The figure shows three views and two pictorial views of one solid part (mm, origin at its lowest corner). Answer the questions. A direction names the side the tool comes from. Round coordinates to 2 decimals unless told otherwise and drop trailing zeros. Order: outer loops, then holes, each group sorted by start corner. A loop starts at its lowest first (then second) coordinate and runs counter-clockwise, first axis right, second up. Notation, with made-up numbers: M 0.5,3.5 L 8.5,3.5 A21 cw 8.5,9.5 Z; hole C 3,-7 d9. An arc over 180 degrees is marked long. Answer as CSV lines item,"result".
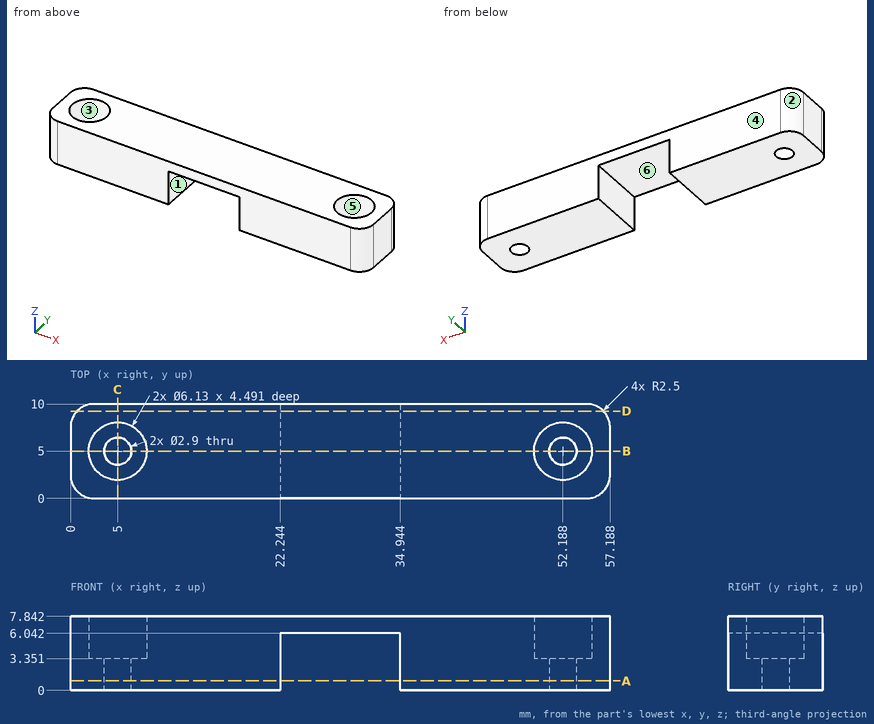
Item 1: A cutting plane is placed at C-C, the plane x = 5. Determine the outline of the cut face in (y, z) (3 decimals).
Ans:
outline,"M 0,0 L 3.55,0 L 3.55,3.351 L 1.935,3.351 L 1.935,7.842 L 0,7.842 Z; M 6.45,0 L 10,0 L 10,7.842 L 8.065,7.842 L 8.065,3.351 L 6.45,3.351 Z"
Item 2: A cutting plane is placed at A-A, the plane z = 1. Determine the outline of the cut face in (x, y).
Ans:
outline,"M 0,2.5 A2.5 ccw 2.5,0 L 22.24,0 L 22.24,10 L 2.5,10 A2.5 ccw 0,7.5 Z; M 34.94,0 L 54.69,0 A2.5 ccw 57.19,2.5 L 57.19,7.5 A2.5 ccw 54.69,10 L 34.94,10 Z; hole C 5,5 d2.9; hole C 52.19,5 d2.9"
Item 3: A cutting plane is placed at D-D, the plane y = 9.25. Determine the outline of the cut face in (x, z) (1 decimal).
Ans:
outline,"M 0.7,0 L 22.2,0 L 22.2,6 L 34.9,6 L 34.9,0 L 56.5,0 L 56.5,7.8 L 0.7,7.8 Z"
Item 4: A cutting plane is placed at B-B, the plane y = 5. Give the number of separate pieces and of enclosed holes in the cut face, and give its area (3 significant figures).
Ans:
separate pieces,"3"
enclosed holes,"0"
area,"297 mm2"
Item 5: Find the intervals of material crossed by probe 1 along X at (y, z) = (5, 1.4); probe 2 along X at (y, z) = (5, 5.35) (1 decimal); probe 3 along X at (y, z) = (5, 6.6) (3 decimals), in increasing order. Write a range as [from, to].
Ans:
probe 1,"[0, 3.55], [6.45, 22.24], [34.94, 50.74], [53.64, 57.19]"
probe 2,"[0, 1.9], [8.1, 22.2], [34.9, 49.1], [55.3, 57.2]"
probe 3,"[0, 1.935], [8.065, 49.123], [55.253, 57.188]"
Item 6: Determine the mould class of the marked faces 4, 5 and 6 for opening direction Y: +Y half, -Y half, draft (parallel to the pull), parting line (faces both ways), or undercut.
Ans:
face 4,"+Y half"
face 5,"undercut"
face 6,"draft"
Item 7: A tool of negligible diameter and unlimited length cuts with its end or side. For the marked faces 1, 2 and 3, from which of +Z, -Z, +X, -X, +Y, -Y can it reach the whole face along a straight path? Write none if from no direction.
Ans:
face 1,"-Z, +Y, -Y"
face 2,"+Z, -Z, -X, +Y"
face 3,"+Z"
Item 8: Flat-ended cylindrical pins translate along their axes: pin 1 (1.8 mm diameter, centred on x = 5.5, y = 6, fed in from +Z); pin 2 (3 mm diameter, centred on y = 8, z = 7, fed in from +X). Find the tip coordinate at first contact, or state that the pin passes through.
Ans:
pin 1,"z = 3.35"
pin 2,"x = 57.19"
